Verification items for this drawing (mm, ordinates from the low corner). A direction names the side the tool comes from. Round coordinates to 2 decimals unless told otherwise and drop trailing zeros. Write each loop counter-clockwise with the first axis right and the second up, starting at its lowest first coordinate (ties: lowest second). Pieces come first, ordered by that corner, then holes. Notation, with made-up numbers: (73.5, 17.5) -> (113.5, 17.5) arc R36 cw to (113.5, 56.5) -> close; hole circle Ø9 at (-16, 35.5). An arc over 180 degrees is marked (long way). Use one line per item in the form item = value. Start each with the question number.
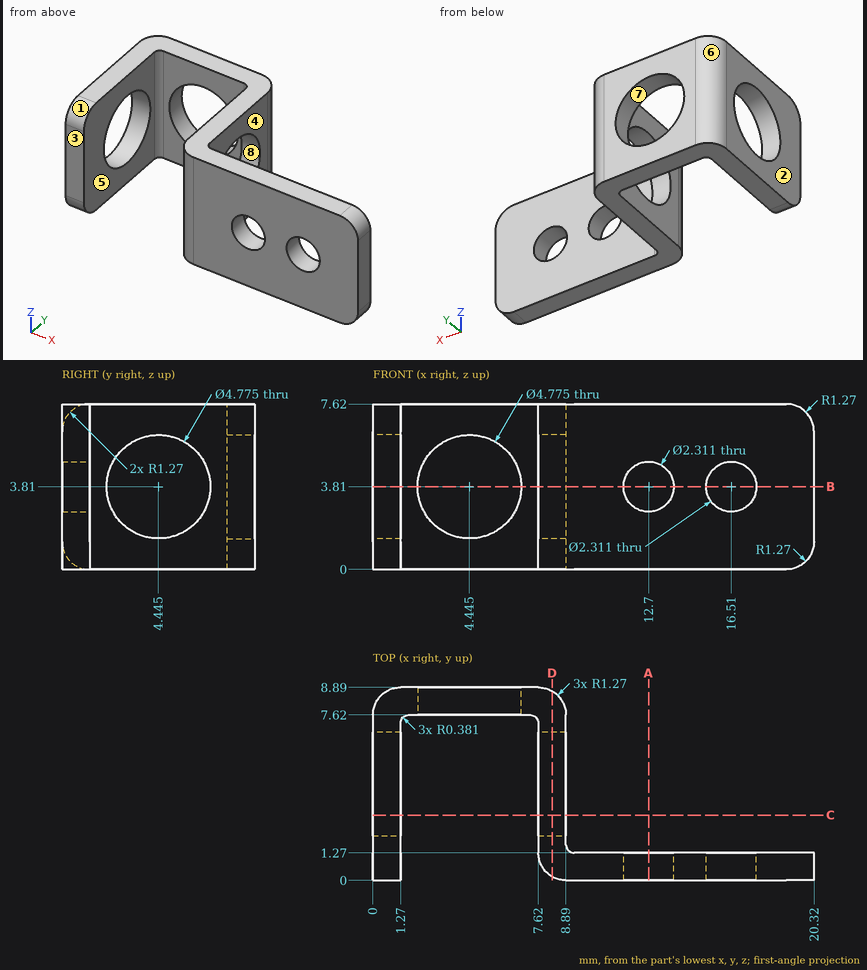
1. Depth check by flat-ended pin: pin 1 (2 mm diameter, centred on y = 6, z = 4, fed in from +X); pin 2 (2.5 mm diameter, centred on x = 17, z = 4.5, fed in from +Y). Enter the tip coordinate at first touch or a pass-through.
2. Sectioned sample at D-D (x = 8.25). Enter the section's corners in (y, z) (1 decimal).
3. Sectioned sample at A-A (x = 12.7). Enter the section's corners in (y, z) (1 decimal).
4. Scan lines: probe 1 along Z at (x, y) = (16.51, 0.75) (1 decimal); probe 2 along X at (y, z) = (7.25, 0.5); probe 3 along X at (y, z) = (1, 3.5). Record each from-to range of solid material in increasing order.
5. Mould release check, pull along X, two halves, no side actions. Record for the marked faces 6, 7 and 8: +X half, -X half, draft (parallel to the pull), parting line (faces both ways), or undercut.
6. Tool access check on the marked faces 1, 2, 3, 4 and 5. Record the directions out of +Z, -Z, +X, -X, +Y, -Y that give a thin tool (end or side, any length) a straight path to the whole face; none if there is none.
7. Sectioned sample at B-B (z = 3.81). Give the number of separate pieces and of enclosed holes in the cut face.
8. Sectioned sample at C-C (y = 3). Enter the section's corners in (x, z).
Returned:
q1.pin_1 = 8.89
q1.pin_2 = 1.27
q2.outline = (0.2, 0) -> (8.7, 0) -> (8.7, 7.6) -> (0.2, 7.6) -> close; hole circle Ø4.8 at (4.4, 3.8)
q3.outline = (0, 0) -> (1.3, 0) -> (1.3, 2.7) -> (0, 2.7) -> close; (0, 5) -> (1.3, 5) -> (1.3, 7.6) -> (0, 7.6) -> close
q4.probe_1 = 0 to 2.7, 5 to 7.6
q4.probe_2 = 0 to 1.27, 7.62 to 8.89
q4.probe_3 = 0 to 1.27, 7.65 to 11.59, 13.81 to 15.4, 17.62 to 20.32
q5.face_6 = -X half
q5.face_7 = undercut
q5.face_8 = draft
q6.face_1 = +Z, -X, -Y
q6.face_2 = +Z, -Z, -X, +Y, -Y
q6.face_3 = +Z, -Z, +X, -X, -Y
q6.face_4 = +Z, -Z, +X, +Y
q6.face_5 = +Z, -Z, -Y
q7.separate_pieces = 6
q7.enclosed_holes = 0
q8.outline = (0, 0) -> (1.27, 0) -> (1.27, 1.91) -> (0, 1.91) -> close; (0, 5.71) -> (1.27, 5.71) -> (1.27, 7.62) -> (0, 7.62) -> close; (7.62, 0) -> (8.89, 0) -> (8.89, 1.91) -> (7.62, 1.91) -> close; (7.62, 5.71) -> (8.89, 5.71) -> (8.89, 7.62) -> (7.62, 7.62) -> close
